Could you check a few things on this model? Use its own coordinates, in mm. Round coordinates to 2 decimals unless told otherwise and drop trailing zeros. Write each loop counter-clockwise with the first axis right and the second up, starting at its lowest first coordinate (ties: lowest second). Pieces come first, ordered by that corner, then holes. Notation, with made-up numbers: (23, 52.5) -> (32, 52.5) arc R29 cw to (32, 90.5) -> close; hole circle Ø5 at (88, -22.5). An arc over 180 degrees is marked (long way). Answer in a Markdown table with one row per item.
from build123d import *

# Parameters (mm, degrees)
SKETCH1_W           = 35
SKETCH1_H           = 80
BOSS_EXTRUDE1_DEPTH = 3
SKETCH2_W           = 9.965503069
SKETCH2_H           = 10
BOSS_EXTRUDE2_DEPTH = 3
SKETCH3_R           = 1
CUT_EXTRUDE2_DEPTH  = 20.272


with BuildPart() as part:
    # Sketch1 → Boss-Extrude1 (new body)
    with BuildSketch(Plane.XY):
        Rectangle(SKETCH1_W, SKETCH1_H)
    extrude(amount=BOSS_EXTRUDE1_DEPTH)

    # Sketch2 → Boss-Extrude2 (add)
    with BuildSketch(Plane.XY):
        with Locations((20.417248466, 0)):
            Rectangle(SKETCH2_W, SKETCH2_H)
    extrude(amount=BOSS_EXTRUDE2_DEPTH)

    # Sketch3 → Cut-Extrude2 (cut)
    with BuildSketch(Plane.XY):
        with Locations(Location((16, 38.5, 0), (0, 0, 180))):
            Circle(SKETCH3_R)
        with Locations(Location((-16, 38.5, 0), (0, 0, 180))):
            Circle(SKETCH3_R)
        with Locations(Location((16, -38.5, 0), (0, 0, 180))):
            Circle(SKETCH3_R)
        with Locations(Location((-16, -38.5, 0), (0, 0, 180))):
            Circle(SKETCH3_R)
    extrude(amount=CUT_EXTRUDE2_DEPTH, mode=Mode.SUBTRACT)


solid = part.part
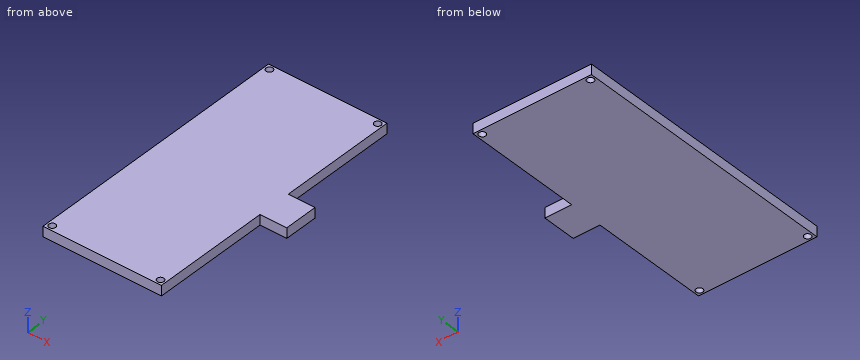
1) Please list where these lines run through material, in increasing order: line 1 (X direction, y = 38.5, z = 2.3); line 2 (Y direction, x = -16, z = 1.65); line 3 (X direction, y = 28, z = 2.6).
Findings:
| item | result |
|---|---|
| line 1 | x = -17.5 to -17, -15 to 15, 17 to 17.5 |
| line 2 | y = -40 to -39.5, -37.5 to 37.5, 39.5 to 40 |
| line 3 | x = -17.5 to 17.5 |
2) Imagine slicing it at D-D, the plane y = -25. Please give me the cut outline in (x, z).
Findings:
| item | result |
|---|---|
| outline | (-17.5, 0) -> (17.5, 0) -> (17.5, 3) -> (-17.5, 3) -> close |
3) Imagine slicing it at C-C, the plane z = 0.45. Please give me the cut outline in (x, y), plus the area to 3 significant figures.
Findings:
| item | result |
|---|---|
| outline | (-17.5, -40) -> (17.5, -40) -> (17.5, -5) -> (25.4, -5) -> (25.4, 5) -> (17.5, 5) -> (17.5, 40) -> (-17.5, 40) -> close; hole circle Ø2 at (-16, -38.5); hole circle Ø2 at (-16, 38.5); hole circle Ø2 at (16, -38.5); hole circle Ø2 at (16, 38.5) |
| area | 2,870 mm^2 |
4) Imagine slicing it at B-B, the plane x = -16. Please give me the cut outline in (y, z), plus the area to 3 significant figures.
Findings:
| item | result |
|---|---|
| outline | (-40, 0) -> (-39.5, 0) -> (-39.5, 3) -> (-40, 3) -> close; (-37.5, 0) -> (37.5, 0) -> (37.5, 3) -> (-37.5, 3) -> close; (39.5, 0) -> (40, 0) -> (40, 3) -> (39.5, 3) -> close |
| area | 228 mm^2 |
5) For pin 1 (1 mm diameter, centred on y = 9, z = 0.5, fed in from +X), with a flat end and sliding along its axis, tell me the tip position at first contact or that it passes through.
Findings:
| item | result |
|---|---|
| pin 1 | stops at x = 17.5 |
6) Imagine slicing it at A-A, the plane y = -38.5. Please give me the cut outline in (x, z), plus the area to 3 significant figures.
Findings:
| item | result |
|---|---|
| outline | (-17.5, 0) -> (-17, 0) -> (-17, 3) -> (-17.5, 3) -> close; (-15, 0) -> (15, 0) -> (15, 3) -> (-15, 3) -> close; (17, 0) -> (17.5, 0) -> (17.5, 3) -> (17, 3) -> close |
| area | 93.0 mm^2 |
